Could you check a few things on this model? Use its own coordinates, in mm. A direction names the side the tool comes from. Coordinates: 2 decimals unless noted, no trailing zeros. Loops run counter-clockwise (first coordinate to the right, second up) from the corner with the lowest first, then second, coordinate; pieces in that order, holes last.
from build123d import *

# Parameters (mm, degrees)
SKETCH_R        = 18
PAD_DEPTH       = 102
SKETCH001_R     = 2.5
POCKET_DEPTH    = 60
SKETCH002_W     = 52.1799999732
SKETCH002_H     = 28
POCKET001_DEPTH = 88.001
SKETCH003_R     = 4.25
POCKET002_DEPTH = 67.1809999732
SKETCH004_R     = 6.8
POCKET003_DEPTH = 6.3
SKETCH005_W     = 11.6986626704
SKETCH005_H     = 15
POCKET004_DEPTH = 28
SKETCH006_W     = 11.6986626704
SKETCH006_H     = 15
POCKET005_DEPTH = 28
SKETCH007_W     = 13
SKETCH007_H     = 52.1799999732
PAD001_DEPTH    = 28


with BuildPart() as part:
    # Sketch → Pad (new body)
    with BuildSketch(Plane.XZ):
        with BuildLine():
            ThreePointArc((-22.8675555461, 17.834654562), (-26.0598687385, -12.7233345209), (-0.0012478604, -28.9999999732))
            Line((-0.0012478604, -28.9999999732), (59, -28.9999999732))
            Line((59, 38.18), (59, -28.9999999732))
            Line((-7, 38.18), (59, 38.18))
            Line((-22.8675555461, 17.834654562), (-7, 38.18))
        make_face()
        Circle(SKETCH_R, mode=Mode.SUBTRACT)
    extrude(amount=PAD_DEPTH)

    # Sketch001 (on Face8 of Pad) → Pocket (cut)
    with BuildSketch(Plane.XZ.offset(102)):
        with Locations((-16.6170093579, 16.6170093579)):
            Circle(SKETCH001_R)
        with Locations((-23.5, 0)):
            Circle(SKETCH001_R)
        with Locations((-16.6170093579, -16.6170093579)):
            Circle(SKETCH001_R)
        with Locations((16.6170093579, -16.6170093579)):
            Circle(SKETCH001_R)
        with Locations((23.5, 0)):
            Circle(SKETCH001_R)
        with Locations((16.6170093579, 16.6170093579)):
            Circle(SKETCH001_R)
    extrude(amount=-POCKET_DEPTH, mode=Mode.SUBTRACT)

    # Sketch002 (on Face7 of Pocket) → Pocket001 (cut, through all)
    with BuildSketch(Plane(origin=(59, 0, 0), x_dir=(0, 0, 1), z_dir=(1, 0, 0))):
        with Locations((-2.9099999866, 88)):
            Rectangle(SKETCH002_W, SKETCH002_H)
        with Locations((-2.9099999866, 14)):
            Rectangle(SKETCH002_W, SKETCH002_H)
    extrude(amount=-POCKET001_DEPTH, mode=Mode.SUBTRACT)

    # Sketch003 (on Face17 of Pocket001) → Pocket002 (cut, through all)
    with BuildSketch(Plane(origin=(0, 0, 38.18), x_dir=(-1, 0, 0), z_dir=(0, 0, 1))):
        with Locations((-39.5284801247, 85.8654773551)):
            Circle(SKETCH003_R)
        with Locations((-4.5184801247, 85.8654773551)):
            Circle(SKETCH003_R)
        with Locations((-39.5284801247, 15.8954773551)):
            Circle(SKETCH003_R)
        with Locations((-4.5184801247, 15.8954773551)):
            Circle(SKETCH003_R)
    extrude(amount=-POCKET002_DEPTH, mode=Mode.SUBTRACT)

    # Sketch004 (on Face9 of Pocket002) → Pocket003 (cut)
    with BuildSketch(Plane(origin=(0, 0, 23.18), x_dir=(1, 0, 0), z_dir=(0, 0, -1))):
        with Locations((4.5184801247, 85.8654773551)):
            Circle(SKETCH004_R)
        with Locations((39.5284801247, 85.8654773551)):
            Circle(SKETCH004_R)
        with Locations((39.5284801247, 15.8954773551)):
            Circle(SKETCH004_R)
        with Locations((4.5184801247, 15.8954773551)):
            Circle(SKETCH004_R)
    extrude(amount=-POCKET003_DEPTH, mode=Mode.SUBTRACT)

    # Sketch005 (on Face18 of Pocket003) → Pocket004 (cut)
    with BuildSketch(Plane.XZ.offset(102)):
        with Locations((-12.8493313352, 30.68)):
            Rectangle(SKETCH005_W, SKETCH005_H)
    extrude(amount=-POCKET004_DEPTH, mode=Mode.SUBTRACT)

    # Sketch006 (on Face17 of Pocket004) → Pocket005 (cut)
    with BuildSketch(Plane(origin=(0, 0, 0), x_dir=(1, 0, 0), z_dir=(0, 1, 0))):
        with Locations((-12.8493313352, -30.68)):
            Rectangle(SKETCH006_W, SKETCH006_H)
    extrude(amount=-POCKET005_DEPTH, mode=Mode.SUBTRACT)

    # Sketch007 (on Face2 of Pocket005) → Pad001 (join)
    with BuildSketch(Plane(origin=(0, -28, 0), x_dir=(1, 0, 0), z_dir=(0, 1, 0))):
        with Locations((24.5, 2.9099999866)):
            Rectangle(SKETCH007_W, SKETCH007_H)
    extrude(amount=PAD001_DEPTH)


solid = part.part
(1) I need wall thicknesses on probe 1 along X at (y, z) = (-11.5, 23.5); probe 2 along Y at (x, z) = (28.5, 4.5); probe 3 along Y at (x, z) = (38.5, -5). Which ranges of each line are inside material? Lowest first, please.
Answers:
probe 1: x = -7 to -0.67, 9.71 to 34.34, 44.72 to 59
probe 2: y = -74 to 0
probe 3: y = -74 to -28
(2) Imagine slicing it at C-C, the plane y = -7.5. Write out the boundary of the cut face in (x, z).
Answers:
outline: (-7, 23.18) - (18, 23.18) - (18, -29) - (31, -29) - (31, 23.18) - (59, 23.18) - (59, 38.18) - (-7, 38.18) - close
(3) We'd pull the mould along Y, two halves only. Please class faces 5 (the face through (2.557, -82.095, 33.891)), 6 (the face through (18, -14, -3)), 7 (the face through (23, -42, 0)): +Y half, -Y half, draft (parallel to the pull), parting line (faces both ways), or undercut.
Answers:
face 5: undercut
face 6: draft
face 7: -Y half
(4) Imagine slicing it at B-B, the plane y = -38.5. Write out the boundary of the cut face in (x, z), and give its area (3 significant figures).
Answers:
outline: (-22.87, 17.83) arc R29 ccw to (0, -29) - (59, -29) - (59, 38.18) - (-7, 38.18) - close; hole circle Ø36 at (0, 0)
area: 4,390 mm2
(5) Which directions (+Z, -Z, +X, -X, +Y, -Y) give clear straight access to the entire face, cutting with the end or side of a thin tool? Please do faces 1 (the face through (1, -13, 29.48)), 2 (the face through (11.2, -13.8, 23.18)), 3 (the face through (26, 0, 19)), 4 (the face through (17, -42, 17)).
Answers:
face 1: -Z
face 2: -Z, -X, +Y
face 3: +Z, -Z, +X, -X, +Y
face 4: -Y
(6) Imagine slicing it at A-A, the plane x = 3. Write out the boundary of the cut face in (y, z), and give its area (3 significant figures).
Answers:
outline: (-102, 23.18) - (-92.49, 23.18) - (-92.49, 29.48) - (-89.83, 29.48) - (-89.83, 38.18) - (-102, 38.18) - close; (-81.9, 29.48) - (-79.24, 29.48) - (-79.24, 23.18) - (-74, 23.18) - (-74, 17.75) - (-28, 17.75) - (-28, 23.18) - (-22.52, 23.18) - (-22.52, 29.48) - (-19.86, 29.48) - (-19.86, 38.18) - (-81.9, 38.18) - close; (-74, -29) - (-28, -29) - (-28, -17.75) - (-74, -17.75) - close; (-11.93, 29.48) - (-9.27, 29.48) - (-9.27, 23.18) - (0, 23.18) - (0, 38.18) - (-11.93, 38.18) - close
area: 1,990 mm2
(7) For pin 1 (11 mm diameter, centred on x = 43, y = -83, fed in from -Z); pin 2 (12 mm diameter, centred on x = 39.53, y = -85.87, fed in from -Z); pin 3 (4.5 mm diameter, centred on x = -16.62, z = -16.62, fed in from -Y), each with a flat end and sliding along its axis, tell me the tip position at first contact or that it passes through.
Answers:
pin 1: stops at z = 23.18
pin 2: stops at z = 29.48
pin 3: stops at y = -42
(8) Imagine slicing it at D-D, the plane x = 23.5. Write out the boundary of the cut face in (y, z), and give its area (3 significant figures).
Answers:
outline: (-102, 23.18) - (-74, 23.18) - (-74, 2.5) - (-42, 2.5) - (-42, -2.5) - (-74, -2.5) - (-74, -29) - (0, -29) - (0, 38.18) - (-102, 38.18) - close
area: 5,230 mm2
